```python
from build123d import *

# Parameters (mm, degrees)
ESQUISSE1_R        = 1.5
BOSS_EXTRU_2_DEPTH = 3


with BuildPart() as part:
    # Esquisse1 → Boss.-Extru.2 (new body)
    with BuildSketch(Plane.XY):
        Polygon((-10.943102451, -5.75), (-2.589352418, 2.864804721), (2.410647582, 2.864804721), (12.46125309, -6.881236984), (9.304151267, -10.136998238), (11.457852448, -12.225435747), (4.496394087, -19.404439681), (2.26460488, -17.24028045), (-0.892496943, -20.496041705), (-10.943102451, -10.75), align=None)
        Circle(ESQUISSE1_R, mode=Mode.SUBTRACT)
        with Locations((-8, -8.25)):
            Circle(ESQUISSE1_R, mode=Mode.SUBTRACT)
    extrude(amount=BOSS_EXTRU_2_DEPTH)


solid = part.part
```
The listing builds one solid part. Answer for the finished solid, in the listing's coordinates (mm). A direction names the side the tool comes from. Round coordinates to 2 decimals unless told otherwise and drop trailing zeros. Loops run counter-clockwise (first coordinate to the right, second up) from the corner with the lowest first, then second, coordinate; pieces in that order, holes last. Notation, with made-up numbers: (-12.5, 89.25) - (11.5, 89.25) arc R15 cw to (11.5, 115.25) - close; hole circle Ø11 at (55, 46.5). An arc over 180 degrees is marked (long way). Return JSON: item names as keys, results as strings. Group by question number.
1. Consider probe 1 along Y at (x, z) = (9.75, 0.85); probe 2 along X at (y, z) = (-17.5, 1.3); probe 3 along Y at (x, z) = (-8, 2). Determine where each line is inside the solid, lowest interval first.
2. The part is cut by section C-C on x = -7.5. Determine the outline of the cut face in (y, z), then the cut area to 3 significant figures.
3. The part is cut by section B-B on y = -8.25. Determine the outline of the cut face in (x, z), then the cut area to 3 significant figures.
4. Each of these flat-tipped pins is pushed along its axis until it touches: P1, Ø8, axis at x = -1, y = -2.5, coming from the -Z side; P2, Ø2.5, axis at x = -8, y = -8.25, coming from the +Z side. Where does it stop, or does it pass through?
5. The part is cut by section D-D on y = -14.25. Determine the outline of the cut face in (x, z).
6. The part is cut by section A-A on z = 1.8. Determine the outline of the cut face in (x, y).
7. Which of the six approach directions +Z, -Z, +X, -X, +Y, -Y give full straight-line access (tool end or side, diameter ignored) to faces 4 (the flat face through (-5.85, -15.69, 1.48)), 5 (the flat face through (10.4, -11.2, 1.5)), 6 (the flat face through (3.4, -18.34, 1.48))?
8. The mould has two halves that part along Y. Classify faces 1 (the cylindrical face through (-8.325, -9.714, 1.479)), 2 (the flat face through (0, 2.865, 1)), 3 (the flat face through (-10.943, -8, 1)): pulls with the +Y half, pulls with the -Y half, needs draft (parallel to the pull), parting line crosses it, or undercut.
Resolved:
{
 "1": {"probe 1": "y = -13.99 to -10.57, -9.68 to -4.25", "probe 2": "x = -3.98 to 2.01, 2.53 to 6.34", "probe 3": "y = -13.6 to -9.75, -6.75 to -2.71"},
 "2": {"outline": "(-14.09, 0) - (-9.66, 0) - (-9.66, 3) - (-14.09, 3) - close; (-6.84, 0) - (-2.2, 0) - (-2.2, 3) - (-6.84, 3) - close", "area": "27.2 mm²"},
 "3": {"outline": "(-10.94, 0) - (-9.5, 0) - (-9.5, 3) - (-10.94, 3) - close; (-6.5, 0) - (11.13, 0) - (11.13, 3) - (-6.5, 3) - close", "area": "57.2 mm²"},
 "4": {"P1": "stops at z = 0", "P2": "passes through"},
 "5": {"outline": "(-7.33, 0) - (9.49, 0) - (9.49, 3) - (-7.33, 3) - close"},
 "6": {"outline": "(-10.94, -10.75) - (-0.89, -20.5) - (2.26, -17.24) - (4.5, -19.4) - (11.46, -12.23) - (9.3, -10.14) - (12.46, -6.88) - (2.41, 2.86) - (-2.59, 2.86) - (-10.94, -5.75) - close; hole circle Ø3 at (-8, -8.25); hole circle Ø3 at (0, 0)"},
 "7": {"face 4": "+Z, -Z, -X, -Y", "face 5": "+Z, -Z, +X", "face 6": "+Z, -Z, -Y"},
 "8": {"face 1": "undercut", "face 2": "pulls with the +Y half", "face 3": "needs draft"}
}
